Check sheet for the modelled part. Datum: model origin and axes. Units: mm. A direction names the side the tool comes from. Round coordinates to 2 decimals unless told otherwise and drop trailing zeros. Loops run counter-clockwise (first coordinate to the right, second up) from the corner with the lowest first, then second, coordinate; pieces in that order, holes last. Notation, with made-up numbers: (-11.5, -22.5) - (47.5, -22.5) arc R28 cw to (47.5, 5.5) - close; hole circle Ø8 at (66, 70.5). An arc over 180 degrees is marked (long way). Answer in a Markdown table with one row per item. Add a question column.
(1) Thickness scan on line 1 along Z through (x, y) = (0, -1.45); line 2 along Z through (x, y) = (-3.75, 0.5); line 3 along Z through (x, y) = (2, -1.75). Record the ranges inside material, lowest first.
(2) Mould release check, pull along Z, two halves, no side actions. Record for faces 4 (the flat face through (2.2, -3.3, 1)), 5 (the cylindrical face through (3.233, -1.341, 35.465)), 6 (the cylindrical face through (-0.54, -2.44, 26.06)): +Z half, -Z half, draft (parallel to the pull), parting line (faces both ways), or undercut.
(3) Cross-section at C-C on z = 11. Enter the section's corners in (x, y), then the cut area to 3 significant figures.
(4) Access from +Z, -Z, +X, -X, +Y, -Y to the whole of each face (thin tool, end or side, straight path). Record for faces 1 (the flat face through (2, -2, 21)), 2 (the cylindrical face through (3.233, -1.341, 10.86)), 3 (the flat face through (0, 0, 38)).
(5) Cross-section at B-B on y = 3. Count the separate pieces of the cut face and the enclosed holes in it, then the cut area to 3 significant figures.
(6) Cross-section at A-A on x = 0. Enter the section's corners in (y, z).
(7) Gauge pin test, flat ends, axial feed: pin 1 (5 mm diameter, centred on x = 1, z = 26, fed in from -Y); pin 2 (2 mm diameter, centred on y = 2.5, z = 25, fed in from -X); pin 3 (1.5 mm diameter, centred on y = 1.5, z = 6, fed in from -X). Record the tip position at first contact, or that the pin passes through.
from build123d import *

# Parameters (mm, degrees)
F0_R     = 3.5
F1_DEPTH = 13
F7_R     = 3.5
F7_R_2   = 2.5
F8_DEPTH = 25
F9_START = 8
F9_DEPTH = 12
F0_R_2   = 5
F3_DEPTH = 1
F5_D     = 1
F5_DEPTH = 5.001
F6_D     = 1
F6_DEPTH = 12
F6_TIP   = 0.3004303095


# Not quite as in the source:
# - a fillet or chamfer that OpenCascade refuses, or shapes differently, is made with other operations: its cross-section is extruded or revolved along the edge and cut away or added


with BuildPart() as f1:
    # F0 (on Top) → F1 (new body)
    with BuildSketch(Plane.XY):
        Circle(F0_R)
    extrude(amount=F1_DEPTH)

    # F7 (on face) → F8 (join)
    with BuildSketch(Plane.XY.offset(13)):
        Circle(F7_R)
        Circle(F7_R_2, mode=Mode.SUBTRACT)
        Circle(F7_R_2)
    extrude(amount=F8_DEPTH)

    # F7 (on face) → F9 (cut)
    with BuildSketch(Plane.XY.offset(13).offset(F9_START)):
        Circle(F7_R)
        Circle(F7_R_2, mode=Mode.SUBTRACT)
    extrude(amount=F9_DEPTH, mode=Mode.SUBTRACT)

    # F2: fillet of radius 2 on 1 edges, made by hand

    # F2_s1 → F2_t2 (revolve)
    with BuildSketch(Plane.XZ):
        with BuildLine():
            ThreePointArc((2.5, 31.2679491924), (2.7679491924, 32.2679491924), (3.5, 33))
            Line((3.5, 33), (2.5, 33))
            Line((2.5, 33), (2.5, 31.2679491924))
        make_face()
    revolve(axis=Axis((0, 0, 33), (0, 0, 1)))

    # F0 (on Top) → F3 (join)
    with BuildSketch(Plane.XY):
        Circle(F0_R_2)
        Circle(F0_R, mode=Mode.SUBTRACT)
    extrude(amount=F3_DEPTH)

    # F5 (through all, one way)
    with BuildSketch(Plane.XZ):
        with Locations((0, 14.4967586048)):
            Circle(F5_D / 2)
    extrude(amount=-F5_DEPTH, mode=Mode.SUBTRACT)

    # F6
    with Locations(Plane(origin=(0, 0, 0), x_dir=(1, 0, 0), z_dir=(0, 1, 0))):
        with Locations((0, -14.4967586048)):
            Hole(F6_D / 2, depth=F6_DEPTH)
            with Locations((0, 0, -(F6_DEPTH + F6_TIP / 2))):  # 118° drill point
                Cone(0, F6_D / 2, F6_TIP, mode=Mode.SUBTRACT)


solid = f1.part
Answers:
| question | item | result |
|---|---|---|
| 1 | line 1 | z = 0 to 14, 15 to 38 |
| 1 | line 2 | z = 0 to 1 |
| 1 | line 3 | z = 0 to 21, 32.05 to 38 |
| 2 | face 4 | +Z half |
| 2 | face 5 | draft |
| 2 | face 6 | undercut |
| 3 | outline | circle Ø7 at (0, 0) |
| 3 | area | 38.5 mm^2 |
| 4 | face 1 | none |
| 4 | face 2 | +Z |
| 4 | face 3 | +Z, +X, -X, +Y, -Y |
| 5 | separate pieces | 2 |
| 5 | enclosed holes | 1 |
| 5 | area | 98.3 mm^2 |
| 6 | outline | (-5, 0) - (5, 0) - (5, 1) - (3.5, 1) - (3.5, 14) - (-3.5, 14) - (-3.5, 1) - (-5, 1) - close; (-3.5, 15) - (3.5, 15) - (3.5, 21) - (2.5, 21) - (2.5, 31.27) arc R2 cw to (3.5, 33) - (3.5, 38) - (-3.5, 38) - (-3.5, 33) arc R2 cw to (-2.5, 31.27) - (-2.5, 21) - (-3.5, 21) - close |
| 7 | pin 1 | stops at y = -2.5 |
| 7 | pin 2 | stops at x = -2 |
| 7 | pin 3 | stops at x = -3.42 |
